```python
from build123d import *

# Parameters (mm, degrees)
CUT_EXTRUDE1_DEPTH      = 38.973
CIRPATTERN1_COUNT       = 6
SKETCH6_W               = 96.85
SKETCH6_H               = 31.496
EXTRUDE1_DEPTH          = 44.45
SKETCH4_R               = 8.001
CUT_EXTRUDE2_DEPTH      = 22.098
HOLE1_D                 = 8.992
HOLE1_DEPTH             = 31.496
LPATTERN1_COUNT         = 2
LPATTERN1_PITCH         = 47.626
SKETCH12_W              = 10
SKETCH12_H              = 10
CUT_EXTRUDE3_DEPTH      = 45.45
CUT_EXTRUDE3_DEPTH_BACK = 45.45
CUT_EXTRUDE4_DEPTH      = 3.175


with BuildPart() as part:
    # Sketch1 → Revolve1 (revolve)
    with BuildSketch(Plane(origin=(0, 0, 0), x_dir=(0, 0, -1), z_dir=(1, 0, 0)), mode=Mode.PRIVATE) as revolve1_sk:
        with BuildLine():
            Line((0, 0), (0, 13.9954))
            Line((0, 13.9954), (-4.6736, 13.9954))
            Line((-4.6736, 13.9954), (-4.6736, 36.487))
            Line((-4.6736, 36.487), (-24.003, 36.487))
            ThreePointArc((-24.003, 36.487), (-24.352925731, 36.556604555), (-24.649578441, 36.754821559))
            Line((-24.649578441, 36.754821559), (-25.867756881, 37.973))
            Line((-25.867756881, 37.973), (-82.3845, 37.973))
            Line((-82.3845, 37.973), (-83.388, 36.9695))
            Line((-83.388, 36.9695), (-96.85, 36.9695))
            Line((-96.85, 36.9695), (-96.85, 0))
            Line((-96.85, 0), (0, 0))
        make_face()
    revolve(revolve1_sk.sketch.rotate(Axis((0, 0, 0), (0, 0, -1)), 90), axis=Axis((0, 0, 0), (0, 0, -1)))  # turned: the seam where the file's is

    # Sketch2 → Cut-Extrude1 (cut, symmetric)
    with BuildSketch(Plane(origin=(0, 0, 0), x_dir=(0, 0, -1), z_dir=(1, 0, 0))):
        with BuildLine():
            Line((-96.85, 34.9885), (-84.15, 34.9885))
            ThreePointArc((-84.15, 34.9885), (-83.790789755, 35.137289755), (-83.642, 35.4965))
            Line((-83.642, 35.4965), (-83.642, 38.1635))
            Line((-83.642, 38.1635), (-96.85, 38.1635))
            Line((-96.85, 38.1635), (-96.85, 34.9885))
        make_face()
    cut_extrude1 = extrude(amount=CUT_EXTRUDE1_DEPTH, both=True, mode=Mode.SUBTRACT)

    # CirPattern1: Cut-Extrude1 ×6 about axis
    cirpattern1_axis = Axis((0, 0, 0), (0, 0, 1))
    for i in range(1, CIRPATTERN1_COUNT):
        add(cut_extrude1.rotate(cirpattern1_axis, i * 360 / CIRPATTERN1_COUNT), mode=Mode.SUBTRACT)

    # Sketch6 → Extrude1 (add, symmetric)
    with BuildSketch(Plane(origin=(0, 0, 0), x_dir=(1, 0, 0), z_dir=(0, 1, 0))):
        with Locations((3.975, -4.902)):
            Rectangle(SKETCH6_W, SKETCH6_H)
    extrude(amount=EXTRUDE1_DEPTH, both=True)

    # Sketch3 → Revolve2 (revolve)
    with BuildSketch(Plane(origin=(0, 0, 0), x_dir=(0, 0, -1), z_dir=(1, 0, 0)), mode=Mode.PRIVATE) as revolve2_sk:
        with BuildLine():
            Line((-112.484, 0), (-112.484, 15.875))
            Line((-112.484, 15.875), (-110.068780748, 24.818188244))
            ThreePointArc((-110.068780748, 24.818188244), (-109.787479807, 25.237840839), (-109.309, 25.4))
            Line((-109.309, 25.4), (-96.85, 25.4))
            Line((-96.85, 25.4), (-96.85, 0))
            Line((-96.85, 0), (-112.484, 0))
        make_face()
    revolve(revolve2_sk.sketch.rotate(Axis((0, 0, 0), (0, 0, 1)), 270), axis=Axis((0, 0, 0), (0, 0, 1)))  # turned: the seam where the file's is

    # Sketch4 → Cut-Extrude2 (cut)
    with BuildSketch(Plane.XY.offset(112.484)):
        Circle(SKETCH4_R)
    extrude(amount=-CUT_EXTRUDE2_DEPTH, mode=Mode.SUBTRACT)

    # Hole1
    with Locations(Plane.XY.offset(20.65)):
        with Locations((-36.5252, 36.5252), (-36.5252, -36.5252), (45.2374, 0)):
            Hole(HOLE1_D / 2, depth=HOLE1_DEPTH)

    # Sketch9 → Cut-Revolve2 (revolve, cut)
    with BuildSketch(Plane(origin=(0, -23.813, 0), x_dir=(-1, 0, 0), z_dir=(0, 1, 0)), mode=Mode.PRIVATE) as cut_revolve2_sk:
        Polygon((-52.4, 7.67), (-52.146, 7.67), (-52.146, 4.368), (-51.6126, 3.8346), (-41.5796, 3.8346), (-41.5796, -0.585), (-52.4, -0.585), align=None)
    cut_revolve2 = revolve(cut_revolve2_sk.sketch.rotate(Axis((52.4, -23.813, -0.585), (-1, 0, 0)), 180), axis=Axis((52.4, -23.813, -0.585), (-1, 0, 0)), mode=Mode.SUBTRACT)  # turned: the seam where the file's is

    # LPattern1: Cut-Revolve2 ×2
    with Locations(*[(0, i * LPATTERN1_PITCH, 0) for i in range(1, LPATTERN1_COUNT)]):
        add(cut_revolve2, mode=Mode.SUBTRACT)

    # Sketch12 → Cut-Extrude3 (cut, two sides)
    with BuildSketch(Plane(origin=(0, 0, 0), x_dir=(0, 0, -1), z_dir=(0, 1, 0))) as cut_extrude3_sk:
        with Locations((-113.445, 25.6375)):
            Rectangle(SKETCH12_W, SKETCH12_H)
        with Locations((-113.445, -25.6375)):
            Rectangle(SKETCH12_W, SKETCH12_H)
    extrude(amount=CUT_EXTRUDE3_DEPTH, mode=Mode.SUBTRACT)
    extrude(cut_extrude3_sk.sketch, amount=-CUT_EXTRUDE3_DEPTH_BACK, mode=Mode.SUBTRACT)

    # Sketch13 → Cut-Revolve4 (revolve, cut)
    with BuildSketch(Plane(origin=(0, 0, 0), x_dir=(0, 0, -1), z_dir=(1, 0, 0)), mode=Mode.PRIVATE) as cut_revolve4_sk:
        Polygon((-112.484, 11.7475), (-111.671, 10.9345), (-112.484, 10.1215), align=None)
    revolve(cut_revolve4_sk.sketch.rotate(Axis((0, 0, 0), (0, 0, 1)), 270), axis=Axis((0, 0, 0), (0, 0, 1)), mode=Mode.SUBTRACT)  # turned: the seam where the file's is

    # Sketch14 → Cut-Extrude4 (cut)
    with BuildSketch(Plane.XY.offset(112.484)):
        with BuildLine():
            Line((-1.5875, -10.818647513), (-1.5875, 10.818647513))
            ThreePointArc((-1.5875, 10.818647513), (0, 10.9345), (1.5875, 10.818647513))
            Line((1.5875, 10.818647513), (1.5875, -10.818647513))
            ThreePointArc((1.5875, -10.818647513), (0, -10.9345), (-1.5875, -10.818647513))
        make_face()
    extrude(amount=-CUT_EXTRUDE4_DEPTH, mode=Mode.SUBTRACT)


solid = part.part
```
Geometry: final body of the model. Coordinates: model frame, mm. A direction names the side the tool comes from. Round coordinates to 2 decimals unless told otherwise and drop trailing zeros. Order: outer loops, then holes, each group sorted by start corner. A loop starts at its lowest first (then second) coordinate and runs counter-clockwise, first axis right, second up. Notation, with made-up numbers: (28.25, 80.25) - (43.25, 80.25) arc R27 ccw to (43.25, 101.25) - close; hole circle Ø1 at (10.25, 1.5). An arc over 180 degrees is marked (long way). Write item = value, one per line. Start each with the question number.
Q1. Ray query, line 1 (Z direction, x = 39, y = -32.5); line 2 (Z direction, x = -20, y = -16.5); line 3 (X direction, y = 14.5, z = 94). Return the intervals inside material, ascending. Write a range as from..to.
Q2. Cut plane A-A on z = 95. Return the cut outline in (x, y).
Q3. Cut plane B-B on z = 61. Return the cut outline in (x, y), and give its area (3 significant figures).
Q4. Pin query (flat end, axial travel): pin 1 (8 mm diameter, centred on y = 23.813, z = -0.585, fed in from +X); pin 2 (2.5 mm diameter, centred on x = -23, y = -1.5, fed in from +Z) (3 decimals); pin 3 (1 mm diameter, centred on y = 33.5, z = 58.5, fed in from -X). Return the tip coordinate at first contact, or that it passes through.
Q5. Pull-direction query (Z, two-part tool) for faces 1 (the flat face through (52.146, 29, 0)), 2 (the flat face through (0, -9, 109.309)), 3 (the flat face through (0, -34.988, 91)); classes: +Z half, -Z half, draft (parallel to the pull), parting line (faces both ways), or undercut.
Q6. Access query for faces 4 (the flat face through (20.638, 0, 110)), 5 (the flat face through (30.217, -17.639, 90.589)), 6 (the flat face through (-30.385, -17.349, 90.589)), 7 (the flat face through (41.58, 24, -1)). Directions: +Z, -Z, +X, -X, +Y, -Y. A direction counts if a zero-diameter tool reaches every point of the face in a straight line with its end or side. Return the directions, or none.
Q7. Cut plane C-C on z = 0.5. Give the number of separate pieces and of enclosed holes in the cut face, and give its area (3 significant figures).
Outcome:
q1.line_1 = -10.85..20.65
q1.line_2 = -10.85..96.85
q1.line_3 = -32.03..32.03
q2.outline = (-36.27, -7.15) - (-24.33, -27.83) arc R36.97 ccw to (-11.94, -34.99) - (11.94, -34.99) arc R36.97 ccw to (24.33, -27.83) - (36.27, -7.15) arc R36.97 ccw to (36.27, 7.15) - (24.33, 27.83) arc R36.97 ccw to (11.94, 34.99) - (-11.94, 34.99) arc R36.97 ccw to (-24.33, 27.83) - (-36.27, 7.15) arc R36.97 ccw to start; hole circle Ø16 at (0, 0)
q3.outline = circle Ø75.95 at (0, 0)
q3.area = 4,530 mm^2
q4.pin_1 = 41.58
q4.pin_2 = 108.445
q4.pin_3 = -18.79
q5.face_1 = undercut
q5.face_2 = +Z half
q5.face_3 = draft
q6.face_4 = +Z, +X, +Y, -Y
q6.face_5 = +Z, +X, -Y
q6.face_6 = +Z, -X, -Y
q6.face_7 = +X
q7.separate_pieces = 1
q7.enclosed_holes = 3
q7.area = 8,230 mm^2
